from build123d import *

# Parameters (mm, degrees)
EXTRUDE_1_DEPTH        = 5
FILLET_1_R             = 10
FILLET_2_R             = 2
HOLE_WIZARD_M2_1_D     = 1.6
HOLE_WIZARD_M2_1_DEPTH = 4
HOLE_WIZARD_M2_1_TIP   = 0.480688495
HOLE_WIZARD_M3_1_D     = 3.4
HOLE_WIZARD_M3_1_DEPTH = 5.6
HOLE_WIZARD_M3_1_TIP   = 1.021463052


with BuildPart() as part:
    # 스케치1 → 보스-돌출1 (new body)
    with BuildSketch(Plane.XY):
        Polygon((-1.5, 13.5), (-1.5, 9.5), (4.5, 9.5), (4.5, 13.5), (20, 13.5), (20, -13.5), (-20, -13.5), (-20, 13.5), align=None)
    extrude(amount=EXTRUDE_1_DEPTH)

    # 필렛1
    fillet_1_edges = [part.edges().sort_by_distance(p)[0] for p in [
        (-20, 13.5, 2.5),
        (20, 13.5, 2.5),
    ]]
    fillet(fillet_1_edges, radius=FILLET_1_R)

    # 필렛2
    fillet_2_edges = [part.edges().sort_by_distance(p)[0] for p in [
        (20, -5, 0),
        (-20, -5, 0),
        (7.25, 13.5, 0),
        (17.071067812, 10.571067812, 0),
        (-17.071067812, 10.571067812, 0),
        (-5.75, 13.5, 0),
    ]]
    fillet(fillet_2_edges, radius=FILLET_2_R)

    # M2 나사 구멍1
    with Locations(Plane(origin=(0, -13.5, 0), x_dir=(-1, 0, 0), z_dir=(0, -1, 0))):
        with Locations((12.5, -3), (0, -3), (-12.5, -3)):
            Hole(HOLE_WIZARD_M2_1_D / 2, depth=HOLE_WIZARD_M2_1_DEPTH)
            with Locations((0, 0, -(HOLE_WIZARD_M2_1_DEPTH + HOLE_WIZARD_M2_1_TIP / 2))):  # 118° drill point
                Cone(0, HOLE_WIZARD_M2_1_D / 2, HOLE_WIZARD_M2_1_TIP, mode=Mode.SUBTRACT)

    # M3 여유 구멍1
    with Locations(Plane(origin=(0, 0, 0), x_dir=(-1, 0, 0), z_dir=(0, 0, -1))):
        with Locations((-13.3, -1.5), (-9.3, 2.5), (-5.3, -1.5), (-9.3, -5.5)):
            Hole(HOLE_WIZARD_M3_1_D / 2, depth=HOLE_WIZARD_M3_1_DEPTH)
            with Locations((0, 0, -(HOLE_WIZARD_M3_1_DEPTH + HOLE_WIZARD_M3_1_TIP / 2))):  # 118° drill point
                Cone(0, HOLE_WIZARD_M3_1_D / 2, HOLE_WIZARD_M3_1_TIP, mode=Mode.SUBTRACT)


solid = part.part
Can you work these out from the model? Positions are in its coordinate system, mm. A direction names the side the tool comes from. Round coordinates to 2 decimals unless told otherwise and drop trailing zeros. Write each loop counter-clockwise with the first axis right and the second up, starting at its lowest first coordinate (ties: lowest second). Pieces come first, ordered by that corner, then holes. Notation, with made-up numbers: M 85.5,19.25 L 137.5,19.25 A23 ccw 137.5,43.25 Z; hole C -31,10 d7. An arc over 180 degrees is marked long. Use a Markdown table: item, result.
Item 1: I want a section at D-D (z = 0.4). List the corners of the cut face in (x, y) for me, and give its area (3 significant figures).
Found:
| item | result |
|---|---|
| outline | M -19.2,-13.5 L 19.2,-13.5 L 19.2,3.5 A9.2 ccw 10,12.7 L 4.5,12.7 L 4.5,9.5 L -1.5,9.5 L -1.5,12.7 L -10,12.7 A9.2 ccw -19.2,3.5 Z; hole C 5.3,-1.5 d3.4; hole C 9.3,-5.5 d3.4; hole C 9.3,2.5 d3.4; hole C 13.3,-1.5 d3.4 |
| area | 914 mm2 |
Item 2: If I drill on line 1 along X through (y, z) = (-11.7, 3); line 2 along Y through (x, z) = (9.3, 2.85); line 3 along X through (y, z) = (-2.75, 1.6), over which ranges is the centre line in solid material (lowest first)? Write a range as [from, to].
Found:
| item | result |
|---|---|
| line 1 | x = [-20, -13.3], [-11.7, -0.8], [0.8, 11.7], [13.3, 20] |
| line 2 | y = [-13.5, -7.2], [-3.8, 0.8], [4.2, 13.5] |
| line 3 | x = [-19.96, 4.15], [6.45, 12.15], [14.45, 19.96] |
Item 3: I want a section at A-A (y = -5.5). List the corners of the cut face in (x, z) for me.
Found:
| item | result |
|---|---|
| outline | M -20,2 A2 ccw -18,0 L 7.6,0 L 7.6,5 L -20,5 Z; M 11,0 L 18,0 A2 ccw 20,2 L 20,5 L 11,5 Z |
Item 4: I want a section at C-C (y = -1.5). List the corners of the cut face in (x, z) for me.
Found:
| item | result |
|---|---|
| outline | M -20,2 A2 ccw -18,0 L 3.6,0 L 3.6,5 L -20,5 Z; M 7,0 L 11.6,0 L 11.6,5 L 7,5 Z; M 15,0 L 18,0 A2 ccw 20,2 L 20,5 L 15,5 Z |
Item 5: I want a section at B-B (x = 5.3). List the corners of the cut face in (y, z) for me.
Found:
| item | result |
|---|---|
| outline | M -13.5,0 L -3.2,0 L -3.2,5 L -13.5,5 Z; M 0.2,0 L 11.5,0 A2 ccw 13.5,2 L 13.5,5 L 0.2,5 Z |
Item 6: For pin 1 Ø2 at (x, y) = (9.3, 2.5) entering from -Z; pin 2 Ø2.5 at (x, z) = (1, 2.5) entering from +Y; pin 3 Ø1.5 at (y, z) = (5.5, 1.5) entering from -X; pin 4 Ø1.4 at (x, z) = (-12.5, 3) entering from -Y, each with a flat end and sliding along its axis, tell me the tip position at first contact or that it passes through.
Found:
| item | result |
|---|---|
| pin 1 | passes through |
| pin 2 | stops at y = 9.5 |
| pin 3 | stops at x = -19.9 |
| pin 4 | stops at y = -9.44 |
Item 7: Which directions (+Z, -Z, +X, -X, +Y, -Y) give clear straight access to the entire face, cutting with the end or side of a thin tool? Please do faces 4 (the face through (-19.4, -4.88, 0.57)), 5 (the face through (1, 9.5, 2)), 6 (the face through (11.87, -11.47, 3.49)).
Found:
| item | result |
|---|---|
| face 4 | -Z, -X, +Y, -Y |
| face 5 | +Z, -Z, +Y |
| face 6 | -Y |
Item 8: We'd pull the mould along Z, two halves only. Please class faces 1 (the face through (4.5, 11, 2)), 2 (the face through (-0.17, -11.47, 3.78)), 3 (the face through (7.29, 12.9, 0.57)): released by +Z, released by -Z, zero draft, split by the parting line, or undercut.
Found:
| item | result |
|---|---|
| face 1 | zero draft |
| face 2 | undercut |
| face 3 | released by -Z |
